Model file for the job. Use its own axes, mm. A direction names the side the tool comes from. Coordinates: 2 decimals unless noted, no trailing zeros. Loops run counter-clockwise (first coordinate to the right, second up) from the corner with the lowest first, then second, coordinate; pieces in that order, holes last. Notation, with made-up numbers: M 13,20.25 L 41,20.25 A16 ccw 41,31.25 Z; hole C 82.5,50.25 d5. An arc over 180 degrees is marked long. One line per question, with ' | ' between items. Start each with the question number.
```python
from build123d import *

# Parameters (mm, degrees)
ESBO_O1_W                = 4
ESBO_O1_H                = 4.25
ESBO_O2_R                = 2.5
RESSALTO_EXTRUS_O1_DEPTH = 12
CORTE_EXTRUS_O1_DEPTH    = 2.5
CHANFRO1_SIZE            = 0.5
FILETE1_R                = 0.2
SKETCH1_R                = 0.25
CUT_EXTRUDE1_DEPTH       = 0.2


with BuildPart() as part:
    # Esboço1 → Revolução1 (revolve)
    with BuildSketch(Plane(origin=(0, 0, 0), x_dir=(-1, 0, 0), z_dir=(0, 0, -1)), mode=Mode.PRIVATE) as revolu_o1_sk:
        with Locations((-2, 2.125)):
            Rectangle(ESBO_O1_W, ESBO_O1_H)
    revolve(revolu_o1_sk.sketch.rotate(Axis((4, 0, 0), (-1, 0, 0)), 270), axis=Axis((4, 0, 0), (-1, 0, 0)))

    # Esboço2 → Ressalto-extrusão1 (add)
    with BuildSketch(Plane(origin=(4, 0, 0), x_dir=(0, 0, -1), z_dir=(1, 0, 0))):
        with Locations((0.4, 0)):
            Circle(ESBO_O2_R)
    extrude(amount=RESSALTO_EXTRUS_O1_DEPTH)

    # Esboço3 → Corte-extrusão1 (cut)
    with BuildSketch(Plane.ZY):
        Polygon((0, -2.357898499), (2.042, -1.17894925), (2.042, 1.17894925), (0, 2.357898499), (-2.042, 1.17894925), (-2.042, -1.17894925), align=None)
    extrude(amount=-CORTE_EXTRUS_O1_DEPTH, mode=Mode.SUBTRACT)

    # Esboço4 → Corte-Revolução1 (revolve, cut)
    with BuildSketch(Plane.XY, mode=Mode.PRIVATE) as corte_revolu_o1_sk:
        Polygon((2.5, 2.042), (2.5, 0), (3.67894925, 0), align=None)
    revolve(corte_revolu_o1_sk.sketch.rotate(Axis((2.5, 0, 0), (1, 0, 0)), 90), axis=Axis((2.5, 0, 0), (1, 0, 0)), mode=Mode.SUBTRACT)

    # Chanfro1
    chanfro1_edges = [part.edges().sort_by_distance(p)[0] for p in [
        (0, 0, -4.25),
        (16, 0, 2.1),
    ]]
    chamfer(chanfro1_edges, length=CHANFRO1_SIZE)

    # Filete1
    filete1_edges = [part.edges().sort_by_distance(p)[0] for p in [
        (4, 0, 2.1),
    ]]
    fillet(filete1_edges, radius=FILETE1_R)

    # Sketch1 → Cut-Extrude1 (cut)
    with BuildSketch(Plane.ZY):
        with Locations((2.8, 0)):
            Circle(SKETCH1_R)
    extrude(amount=-CUT_EXTRUDE1_DEPTH, mode=Mode.SUBTRACT)


solid = part.part
```
(1) Pin check, flat tip, straight feed: P1, Ø5, axis at x = 3.5, y = 3.5, coming from the +Z side. Stop position of the tip, or through.
(2) Band-saw the part on A-A on x = 5.25. Write the cut outline in (y, z).
(3) 3-axis set-ups, long thin cutter, end or side, ignore diameter. For faces 1 (the face through (4, -2, 2)), 2 (the face through (1.232, 1.76, 1.035)), 3 (the face through (2.226, 4.214, -0.553)): which of +Z, -Z, +X, -X, +Y, -Y reach the whole face in a straight line?
(4) Two-plate mould, pull along Y, no slides. Class faces 4 (the face through (1, 0, 2.042)), 5 (the face through (9.771, 0.751, -2.785)), 6 (the face through (1.232, 1.777, -1.007)), 7 (the face through (0, -2, -2)): pulls with the +Y half, pulls with the -Y half, needs draft (parallel to the pull), parting line crosses it, or undercut.
(5) Drill centre lines: line 1 (Z direction, x = 1.75, y = 1.75); line 2 (Z direction, x = 2, y = 1.25); line 3 (X direction, y = 0, z = 3). Where is each one in solid material? Low to high. Write a range as [from, to].
(6) Band-saw the part on B-B on x = 3.25. Write the cut outline in (y, z).
Computed values:
1) P1: z = 4.13
2) outline: C 0,-0.4 d5
3) face 1: +X | face 2: -X | face 3: +X, -X
4) face 4: undercut | face 5: parting line crosses it | face 6: undercut | face 7: needs draft
5) line 1: [-3.87, -1.05], [1.05, 3.87] | line 2: [-4.06, -1.92], [1.92, 4.06] | line 3: [0.2, 4]
6) outline: C 0,0 d8.5; hole C 0,0 d1.49
